For this review, take the finished solid that the model builds, in its own axes (mm). Give positions to 0.01 mm unless a question says otherwise; leave off trailing zeros. Write each loop counter-clockwise with the first axis right and the second up, starting at its lowest first coordinate (ties: lowest second). Pieces come first, ordered by that corner, then holes. Notation, with made-up numbers: (26, 58) -> (55, 58) arc R20 ccw to (55, 87) -> close; hole circle Ø9 at (55.25, 41.5). An arc over 180 degrees is marked (long way). Answer as CSV lines item,"result".
```python
from build123d import *

# Parameters (mm, degrees)
BOSS_EXTRU_2_REACH             = 10
ESQUISSE3_W                    = 7.493865796
ESQUISSE3_H                    = 2.51391664
BOSS_EXTRU_2_DIRECTION_2_DEPTH = 5


with BuildPart() as part:
    # Esquisse1 → R_volution2 (revolve)
    with BuildSketch(Plane(origin=(0, 0, 0), x_dir=(0, 0, -1), z_dir=(1, 0, 0)), mode=Mode.PRIVATE) as r_volution2_sk:
        with BuildLine():
            Line((0, 7), (0, 8))
            Line((0, 8), (1, 7.681145748))
            ThreePointArc((1, 7.681145748), (4.273107431, 5.101924854), (5.903887779, 1.267062649))
            Line((5.903887779, 1.267062649), (5.963189718, 0.268822557))
            Line((5.963189718, 0.268822557), (5, 0))
            ThreePointArc((5, 0), (3.621627687, 4.301162634), (0, 7))
        make_face()
    revolve(r_volution2_sk.sketch.rotate(Axis((0, 19.327032319, 0), (0, -1, 0)), 180), axis=Axis((0, 19.327032319, 0), (0, -1, 0)))  # turned: the seam where the file's is

    # Esquisse3 → Boss.-Extru.2 (add, up to next)
    with BuildSketch(Plane(origin=(0, 8, 0), x_dir=(-1, 0, 0), z_dir=(0, -1, 0)), mode=Mode.PRIVATE) as boss_extru_2_sk1:
        Rectangle(ESQUISSE3_W, ESQUISSE3_H)
    boss_extru_2_tool1 = extrude(boss_extru_2_sk1.sketch, amount=BOSS_EXTRU_2_REACH, mode=Mode.PRIVATE) - part.part
    add(boss_extru_2_tool1.solids().sort_by_distance((0, 8, 0))[0])

    # Esquisse3 → Boss.-Extru.2 direction 2 (add)
    with BuildSketch(Plane(origin=(0, 8, 0), x_dir=(-1, 0, 0), z_dir=(0, -1, 0))):
        Rectangle(ESQUISSE3_W, ESQUISSE3_H)
    extrude(amount=-BOSS_EXTRU_2_DIRECTION_2_DEPTH)


solid = part.part
```
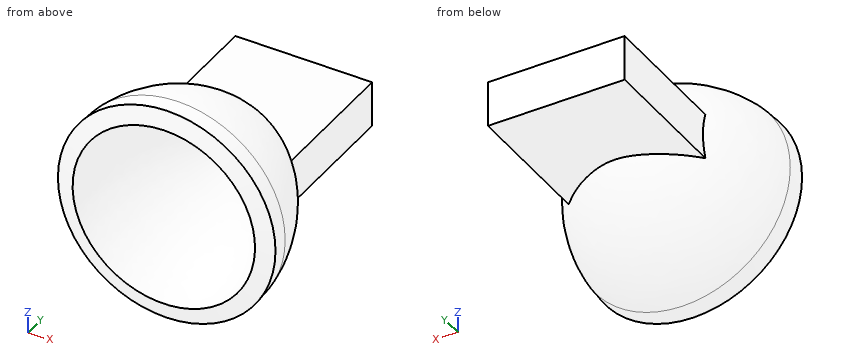
Q1. Add section A-A (y = 8.75). Write out the cut boundary in (x, z).
Answer block:
outline,"(-3.75, -1.26) -> (3.75, -1.26) -> (3.75, 1.26) -> (-3.75, 1.26) -> close"
Q2. Clearance check with flat-ended pins moving along their axes: pin 1 (3 mm diameter, centred on x = 2.5, y = 10, fed in from -Z); pin 2 (1.3 mm diameter, centred on y = 9.5, z = 0.5, fed in from +X); pin 3 (1.5 mm diameter, centred on x = -0.5, z = 3, fed in from +Y); pin 4 (1 mm diameter, centred on y = 11.5, z = 2.5, fed in from +X). State where each tip first meets the part, or that it passes through.
Answer block:
pin 1,"stops at z = -1.26"
pin 2,"stops at x = 3.75"
pin 3,"stops at y = 6.97"
pin 4,"passes through"
Q3. To check wall thickness, follow probe 1 along Z at (x, y) = (-1.75, 7.25); probe 2 along Z at (x, y) = (-0.5, 1); probe 3 along X at (y, z) = (5.5, 2.25). State the ranges of each line that lie inside material, in increasing order. Write a range as [from, to].
Answer block:
probe 1,"z = [-1.26, 1.26]"
probe 2,"z = [-5.9, -4.91], [4.91, 5.9]"
probe 3,"x = [-3.25, -1.2], [1.2, 3.25]"
